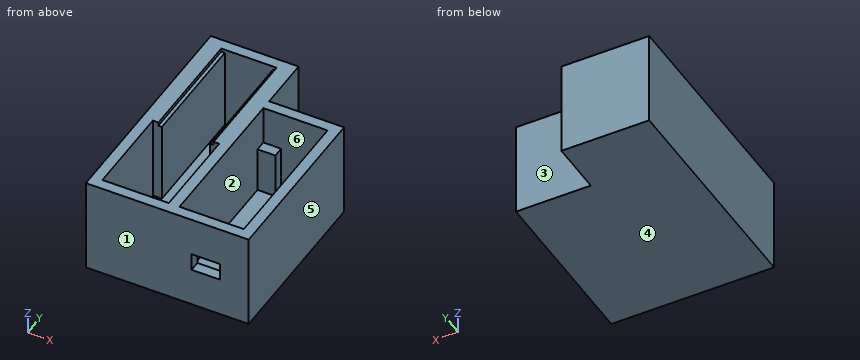
from build123d import *

# Parameters (mm, degrees)
SKETCH1_W            = 1
SKETCH1_H            = 32.4
SKETCH1_W_2          = 13.5
SKETCH1_W_3          = 1.55
SKETCH1_W_4          = 3
SKETCH1_H_2          = 3
SKETCH1_W_5          = 18.6
SKETCH1_H_3          = 26
BOSS_EXTRUDE1_DEPTH  = 3
SKETCH1_5_W          = 3
SKETCH1_5_H          = 3
SKETCH1_5_W_2        = 1
SKETCH1_5_H_2        = 32.4
SKETCH1_5_W_3        = 1.55
BOSS_EXTRUDE2_DEPTH  = 26
BOSS_EXTRUDE4_DEPTH  = 35
SKETCH1_8_W          = 1.55
SKETCH1_8_H          = 32.4
SKETCH1_8_W_2        = 3
SKETCH1_8_H_2        = 3
BOSS_EXTRUDE5_DEPTH  = 27
BOSS_EXTRUDE6_DEPTH  = 3
SKETCH2_3_W          = 3
SKETCH2_3_H          = 3
SKETCH2_3_W_2        = 5
BOSS_EXTRUDE7_DEPTH  = 2
SKETCH2_4_W          = 8
SKETCH2_4_H          = 3
BOSS_EXTRUDE8_DEPTH  = 11
SKETCH2_5_W          = 3
SKETCH2_5_H          = 3
BOSS_EXTRUDE9_DEPTH  = 27
SKETCH5_W            = 30.618778274
SKETCH5_H            = 3
SKETCH5_W_2          = 2.981221726
SKETCH5_H_2          = 60.4
SKETCH5_H_3          = 54.4
BOSS_EXTRUDE11_DEPTH = 3
SKETCH5_5_W          = 30.618778274
SKETCH5_5_H          = 54.4
CUT_EXTRUDE3_DEPTH   = 3
SKETCH5_6_W          = 30.618778274
SKETCH5_6_H          = 3
SKETCH5_6_W_2        = 2.981221726
SKETCH5_6_H_2        = 60.4
BOSS_EXTRUDE12_DEPTH = 27
SKETCH6_W            = 30.618778274
SKETCH6_H            = 47.4
BOSS_EXTRUDE13_DEPTH = 3
SKETCH7_W            = 24.6
SKETCH7_H            = 8
CUT_EXTRUDE4_DEPTH   = 3
SKETCH8_W            = 11
SKETCH8_H            = 3
BOSS_EXTRUDE14_DEPTH = 8
SKETCH2_6_W          = 5
SKETCH2_6_H          = 3
SKETCH2_6_W_2        = 3
BOSS_EXTRUDE15_DEPTH = 16
SKETCH9_W            = 36.6
SKETCH9_H            = 3
BOSS_EXTRUDE16_DEPTH = 15
SKETCH10_W           = 18.8
SKETCH10_H           = 11.60179211
CUT_EXTRUDE5_DEPTH   = 15
BOSS_EXTRUDE17_DEPTH = 3
BOSS_EXTRUDE18_DEPTH = 3
SKETCH13_W           = 33.6
SKETCH13_H           = 60.4
CUT_EXTRUDE6_DEPTH   = 70
CUT_EXTRUDE7_DEPTH   = 70


with BuildPart() as part:
    # Sketch1 → Boss-Extrude1 (new body)
    with BuildSketch(Plane.XY):
        with Locations((-16.55, 42.2)):
            Rectangle(SKETCH1_W, SKETCH1_H)
        with Locations((-9.3, 42.2)):
            Rectangle(SKETCH1_W_2, SKETCH1_H)
        with Locations((-2.05, 42.2)):
            Rectangle(SKETCH1_W, SKETCH1_H)
        with Locations((-0.775, 42.2)):
            Rectangle(SKETCH1_W_3, SKETCH1_H)
        with Locations((-17.825, 42.2)):
            Rectangle(SKETCH1_W_3, SKETCH1_H)
        Polygon((-21.6, 0), (-18.6, 0), (-18.6, 26), (-18.6, 58.4), (-21.6, 58.4), align=None)
        with Locations((-20.1, 59.9)):
            Rectangle(SKETCH1_W_4, SKETCH1_H_2)
        Polygon((-1.55, 58.4), (0, 58.4), (0, 61.4), (-18.6, 61.4), (-18.6, 58.4), (-17.05, 58.4), (-16.05, 58.4), (-2.55, 58.4), align=None)
        with Locations((1.5, 59.9)):
            Rectangle(SKETCH1_W_4, SKETCH1_H_2)
        Polygon((0, 26), (0, 0), (3, 0), (3, 58.4), (0, 58.4), align=None)
        with Locations((-9.3, 13)):
            Rectangle(SKETCH1_W_5, SKETCH1_H_3)
        Polygon((-21.6, -3), (-21.6, 0), (-18.6, 0), (0, 0), (3, 0), (3, -3), align=None)
    extrude(amount=BOSS_EXTRUDE1_DEPTH)

    # Sketch1_5 → Boss-Extrude2 (add)
    with BuildSketch(Plane.XY):
        with Locations((-20.1, 59.9)):
            Rectangle(SKETCH1_5_W, SKETCH1_5_H)
        Polygon((-1.55, 58.4), (0, 58.4), (0, 61.4), (-18.6, 61.4), (-18.6, 58.4), (-17.05, 58.4), (-16.05, 58.4), (-2.55, 58.4), align=None)
        with Locations((-2.05, 42.2)):
            Rectangle(SKETCH1_5_W_2, SKETCH1_5_H_2)
        with Locations((-0.775, 42.2)):
            Rectangle(SKETCH1_5_W_3, SKETCH1_5_H_2)
        with Locations((-16.55, 42.2)):
            Rectangle(SKETCH1_5_W_2, SKETCH1_5_H_2)
        with Locations((-17.825, 42.2)):
            Rectangle(SKETCH1_5_W_3, SKETCH1_5_H_2)
        Polygon((-21.6, 0), (-18.6, 0), (-18.6, 26), (-18.6, 58.4), (-21.6, 58.4), align=None)
        with Locations((1.5, 59.9)):
            Rectangle(SKETCH1_5_W, SKETCH1_5_H)
        Polygon((0, 26), (0, 0), (3, 0), (3, 58.4), (0, 58.4), align=None)
        Polygon((-21.6, -3), (-21.6, 0), (-18.6, 0), (0, 0), (3, 0), (3, -3), align=None)
    extrude(amount=BOSS_EXTRUDE2_DEPTH)

    # Sketch1_7 → Boss-Extrude4 (add)
    with BuildSketch(Plane.XY):
        Polygon((-21.6, -3), (-21.6, 0), (-18.6, 0), (0, 0), (3, 0), (3, -3), align=None)
    extrude(amount=BOSS_EXTRUDE4_DEPTH)

    # Sketch1_8 → Boss-Extrude5 (add)
    with BuildSketch(Plane.XY):
        with Locations((-17.825, 42.2)):
            Rectangle(SKETCH1_8_W, SKETCH1_8_H)
        Polygon((-21.6, 0), (-18.6, 0), (-18.6, 26), (-18.6, 58.4), (-21.6, 58.4), align=None)
        with Locations((-20.1, 59.9)):
            Rectangle(SKETCH1_8_W_2, SKETCH1_8_H_2)
        Polygon((-1.55, 58.4), (0, 58.4), (0, 61.4), (-18.6, 61.4), (-18.6, 58.4), (-17.05, 58.4), (-16.05, 58.4), (-2.55, 58.4), align=None)
        with Locations((1.5, 59.9)):
            Rectangle(SKETCH1_8_W_2, SKETCH1_8_H_2)
        Polygon((0, 26), (0, 0), (3, 0), (3, 58.4), (0, 58.4), align=None)
        with Locations((-0.775, 42.2)):
            Rectangle(SKETCH1_8_W, SKETCH1_8_H)
        Polygon((-21.6, -3), (-21.6, 0), (-18.6, 0), (0, 0), (3, 0), (3, -3), align=None)
    extrude(amount=BOSS_EXTRUDE5_DEPTH)

    # Sketch2 → Boss-Extrude6 (add)
    with BuildSketch(Plane(origin=(0, 0, 0), x_dir=(-1, 0, 0), z_dir=(0, 0, -1))):
        Polygon((-8, 0), (-6, 0), (-6, 3), (-3, 3), (-3, 40.2), (-8, 40.2), (-8, 43.2), (-16, 43.2), (-16, 40.2), (-21, 40.2), (-21, 3), (-18, 3), (-18, 0), (-16, 0), align=None)
    extrude(amount=-BOSS_EXTRUDE6_DEPTH)

    # Sketch2_3 → Boss-Extrude7 (add)
    with BuildSketch(Plane(origin=(0, 0, 0), x_dir=(-1, 0, 0), z_dir=(0, 0, -1))):
        with Locations((-4.5, 1.5)):
            Rectangle(SKETCH2_3_W, SKETCH2_3_H)
        Polygon((-3, -3), (-3, 0), (-6, 0), (-8, 0), (-8, -3), align=None)
        with Locations((-19.5, 1.5)):
            Rectangle(SKETCH2_3_W, SKETCH2_3_H)
        Polygon((-21, -3), (-16, -3), (-16, 0), (-18, 0), (-21, 0), align=None)
        with Locations((-22.5, -1.5)):
            Rectangle(SKETCH2_3_W, SKETCH2_3_H)
        Polygon((-8, 43.2), (-3, 43.2), (-3, 46.2), (-24, 46.2), (-24, 43.2), (-24, 0), (-21, 0), (-21, 3), (-21, 40.2), (-21, 43.2), (-16, 43.2), align=None)
        with Locations((-18.5, 41.7)):
            Rectangle(SKETCH2_3_W_2, SKETCH2_3_H)
        with Locations((-5.5, 41.7)):
            Rectangle(SKETCH2_3_W_2, SKETCH2_3_H)
    extrude(amount=-BOSS_EXTRUDE7_DEPTH)

    # Sketch2_4 → Boss-Extrude8 (add)
    with BuildSketch(Plane(origin=(0, 0, 0), x_dir=(-1, 0, 0), z_dir=(0, 0, -1))):
        with Locations((-12, -1.5)):
            Rectangle(SKETCH2_4_W, SKETCH2_4_H)
    extrude(amount=-BOSS_EXTRUDE8_DEPTH)

    # Sketch2_5 → Boss-Extrude9 (add)
    with BuildSketch(Plane(origin=(0, 0, 0), x_dir=(-1, 0, 0), z_dir=(0, 0, -1))):
        Polygon((-3, -3), (-3, 0), (-6, 0), (-8, 0), (-8, -3), align=None)
        Polygon((-21, -3), (-16, -3), (-16, 0), (-18, 0), (-21, 0), align=None)
        with Locations((-22.5, -1.5)):
            Rectangle(SKETCH2_5_W, SKETCH2_5_H)
        Polygon((-8, 43.2), (-3, 43.2), (-3, 46.2), (-24, 46.2), (-24, 43.2), (-24, 0), (-21, 0), (-21, 3), (-21, 40.2), (-21, 43.2), (-16, 43.2), align=None)
    extrude(amount=-BOSS_EXTRUDE9_DEPTH)

    # Sketch5 → Boss-Extrude11 (add)
    with BuildSketch(Plane(origin=(0, 0, 0), x_dir=(-1, 0, 0), z_dir=(0, 0, -1))):
        with Locations((36.909389137, 55.9)):
            Rectangle(SKETCH5_W, SKETCH5_H)
        with Locations((53.709389137, 27.2)):
            Rectangle(SKETCH5_W_2, SKETCH5_H_2)
        with Locations((36.909389137, -1.5)):
            Rectangle(SKETCH5_W, SKETCH5_H)
        with Locations((36.909389137, 27.2)):
            Rectangle(SKETCH5_W, SKETCH5_H_3)
    extrude(amount=-BOSS_EXTRUDE11_DEPTH)

    # Sketch5_5 → Cut-Extrude3 (cut)
    with BuildSketch(Plane(origin=(0, 0, 0), x_dir=(-1, 0, 0), z_dir=(0, 0, -1))):
        with Locations((36.909389137, 27.2)):
            Rectangle(SKETCH5_5_W, SKETCH5_5_H)
    extrude(amount=-CUT_EXTRUDE3_DEPTH, mode=Mode.SUBTRACT)

    # Sketch5_6 → Boss-Extrude12 (add)
    with BuildSketch(Plane(origin=(0, 0, 0), x_dir=(-1, 0, 0), z_dir=(0, 0, -1))):
        with Locations((36.909389137, 55.9)):
            Rectangle(SKETCH5_6_W, SKETCH5_6_H)
        with Locations((53.709389137, 27.2)):
            Rectangle(SKETCH5_6_W_2, SKETCH5_6_H_2)
        with Locations((36.909389137, -1.5)):
            Rectangle(SKETCH5_6_W, SKETCH5_6_H)
    extrude(amount=-BOSS_EXTRUDE12_DEPTH)

    # Sketch6 → Boss-Extrude13 (add)
    with BuildSketch(Plane.XY.offset(27)):
        with Locations((-36.909389137, 23.7)):
            Rectangle(SKETCH6_W, SKETCH6_H)
    extrude(amount=-BOSS_EXTRUDE13_DEPTH)

    # Sketch7 → Cut-Extrude4 (cut)
    with BuildSketch(Plane.XZ.offset(3)):
        with Locations((-9.3, 31)):
            Rectangle(SKETCH7_W, SKETCH7_H)
    extrude(amount=-CUT_EXTRUDE4_DEPTH, mode=Mode.SUBTRACT)

    # Sketch8 → Boss-Extrude14 (add)
    with BuildSketch(Plane(origin=(8, 0, 0), x_dir=(0, 0, -1), z_dir=(1, 0, 0))):
        with Locations((-21.5, -1.5)):
            Rectangle(SKETCH8_W, SKETCH8_H)
    extrude(amount=BOSS_EXTRUDE14_DEPTH)

    # Sketch2_6 → Boss-Extrude15 (add)
    with BuildSketch(Plane(origin=(0, 0, 0), x_dir=(-1, 0, 0), z_dir=(0, 0, -1))):
        with Locations((-5.5, 41.7)):
            Rectangle(SKETCH2_6_W, SKETCH2_6_H)
        with Locations((-18.5, 41.7)):
            Rectangle(SKETCH2_6_W, SKETCH2_6_H)
        with Locations((-19.5, 1.5)):
            Rectangle(SKETCH2_6_W_2, SKETCH2_6_H)
        with Locations((-4.5, 1.5)):
            Rectangle(SKETCH2_6_W_2, SKETCH2_6_H)
    extrude(amount=-BOSS_EXTRUDE15_DEPTH)

    # Sketch9 → Boss-Extrude16 (add)
    with BuildSketch(Plane.XY.offset(27)):
        with Locations((-36.9, -1.5)):
            Rectangle(SKETCH9_W, SKETCH9_H)
    extrude(amount=BOSS_EXTRUDE16_DEPTH)

    # Sketch10 → Cut-Extrude5 (cut)
    with BuildSketch(Plane(origin=(0, -3, 0), x_dir=(-1, 0, 0), z_dir=(0, -1, 0))):
        with Locations((39.656308117, -34.500896055)):
            Rectangle(SKETCH10_W, SKETCH10_H)
    extrude(amount=-CUT_EXTRUDE5_DEPTH, mode=Mode.SUBTRACT)

    # Sketch11 → Boss-Extrude17 (add)
    with BuildSketch(Plane(origin=(0, -3, 0), x_dir=(-1, 0, 0), z_dir=(0, -1, 0))):
        Polygon((18.6, -42), (18.6, -27), (3.6, -27), align=None)
    extrude(amount=-BOSS_EXTRUDE17_DEPTH)

    # Sketch12 → Boss-Extrude18 (add)
    with BuildSketch(Plane.ZY.offset(55.2)):
        Polygon((27, 0), (42, 0), (27, 15), align=None)
    extrude(amount=-BOSS_EXTRUDE18_DEPTH)

    # Sketch13 → Cut-Extrude6 (cut)
    with BuildSketch(Plane.XY.offset(42)):
        with Locations((-38.4, 27.2)):
            Rectangle(SKETCH13_W, SKETCH13_H)
    extrude(amount=-CUT_EXTRUDE6_DEPTH, mode=Mode.SUBTRACT)

    # Sketch14 → Cut-Extrude7 (cut)
    with BuildSketch(Plane(origin=(0, -3, 0), x_dir=(-1, 0, 0), z_dir=(0, -1, 0))):
        Polygon((3.6, -27), (21.6, -27), (21.6, -42), (18.6, -42), align=None)
    extrude(amount=-CUT_EXTRUDE7_DEPTH, mode=Mode.SUBTRACT)


solid = part.part
Could you check a few things on this model? Use its own coordinates, in mm. Face numbers are marked on the shaded views. A direction names the side the tool comes from. Give positions to 0.01 mm unless a question says otherwise; leave off trailing zeros. Loops run counter-clockwise (first coordinate to the right, second up) from the corner with the lowest first, then second, coordinate; pieces in that order, holes last. Notation, with made-up numbers: (36, 16.5) -> (61, 16.5) arc R15 ccw to (61, 41.5) -> close; hole circle Ø11 at (-1, -23). An arc over 180 degrees is marked (long way). Return JSON: item names as keys, results as strings.
Item 1: If we section it at D-D on y = 42.5: List the corners of the cut face in (x, z) for me, plus the area to 3 significant figures.
Geometry results:
{"outline": "(-21.6, 0) -> (24, 0) -> (24, 27) -> (21, 27) -> (21, 16) -> (16, 16) -> (16, 3) -> (8, 3) -> (8, 16) -> (3, 16) -> (3, 27) -> (-1.55, 27) -> (-1.55, 26) -> (-2.55, 26) -> (-2.55, 3) -> (-16.05, 3) -> (-16.05, 26) -> (-17.05, 26) -> (-17.05, 27) -> (-21.6, 27) -> close", "area": "603 mm²"}
Item 2: Which directions (+Z, -Z, +X, -X, +Y, -Y) give clear straight access to the entire face, cutting with the end or side of a thin tool? Please do the marked faces 1, 2 and 3.
Geometry results:
{"face 1": "+Z, -Z, +X, -X, -Y", "face 2": "+Z", "face 3": "+Z, -Z, +X, +Y"}
Item 3: If we section it at C-C on x = 4: List the corners of the cut face in (y, z) for me, plus the area to 3 significant figures.
Geometry results:
{"outline": "(-3, 0) -> (46.2, 0) -> (46.2, 27) -> (43.2, 27) -> (43.2, 16) -> (40.2, 16) -> (40.2, 3) -> (3, 3) -> (3, 16) -> (0, 16) -> (0, 27) -> (-3, 27) -> close", "area": "370 mm²"}
Item 4: If we section it at A-A on z = 22.75: List the corners of the cut face in (x, y) for me, plus the area to 3 significant figures.
Geometry results:
{"outline": "(-21.6, -3) -> (24, -3) -> (24, 46.2) -> (3, 46.2) -> (3, 61.4) -> (-21.6, 61.4) -> close; hole (-18.6, 0) -> (0, 0) -> (0, 26) -> (-2.55, 26) -> (-2.55, 58.4) -> (-16.05, 58.4) -> (-16.05, 26) -> (-18.6, 26) -> close; hole (3, 0) -> (21, 0) -> (21, 43.2) -> (3, 43.2) -> close", "area": "919 mm²"}
Item 5: We'd pull the mould along X, two halves only. Please class the marked faces 4, 5 and 6: +X half, -X half, draft (parallel to the pull), parting line (faces both ways), or undercut.
Geometry results:
{"face 4": "draft", "face 5": "+X half", "face 6": "undercut"}
Item 6: I need wall thicknesses on L1, parallel to X at y = 31.5, z = 17; L2, parallel to X at y = 0.5, z = 19; L3, parallel to Y at x = 7, z = 22.5. Which ranges of each line are inside material? Lowest first, please. Write a range as from..to.
Geometry results:
{"L1": "x = -21.6..-16.05, -2.55..3, 21..24", "L2": "x = -21.6..-18.6, 0..3, 21..24", "L3": "y = -3..0, 43.2..46.2"}
Item 7: I'm going to push flat-ended pins straight in: pin 1 (1.5 mm diameter, centred on x = 19, y = 1, fed in from +Z); pin 2 (1.5 mm diameter, centred on x = 17, z = 4.5, fed in from +Y); pin 3 (0.8 mm diameter, centred on x = -16.5, y = 49, fed in from +Z). Where does each tip first touch, or does it pass through?
Geometry results:
{"pin 1": "stops at z = 16", "pin 2": "stops at y = 46.2", "pin 3": "stops at z = 26"}
